```python
from build123d import *

# Parameters (mm, degrees)
EXTRUDE1_DEPTH = 101.6
EXTRUDE2_REACH = 180.036
SKETCH2_R      = 27.805675623


with BuildPart() as part:
    # Sketch1 → Extrude1 (new body)
    with BuildSketch(Plane(origin=(0, 0, 0), x_dir=(1, 0, 0), z_dir=(0, 1, 0))):
        Polygon((0, 36.981224411), (0, 0), (42.615353822, 0), (51.897733448, -10.30089681), (80.325021053, -10.30089681), (89.607400679, 0), (132.222754501, 0), (132.222754501, 36.981224411), align=None)
    extrude(amount=-EXTRUDE1_DEPTH)

    # Sketch2 → Extrude2 (add, up to next)
    with BuildSketch(Plane.XY.offset(25.4), mode=Mode.PRIVATE) as extrude2_sk1:
        with Locations((66.111377251, -50.8)):
            Circle(SKETCH2_R)
    extrude2_tool1 = extrude(extrude2_sk1.sketch, amount=-EXTRUDE2_REACH, mode=Mode.PRIVATE) - part.part
    add(extrude2_tool1.solids().sort_by_distance((66.111377, -50.8, 25.4))[0])


solid = part.part
```
Work out the finished part from the listing and answer in its coordinate system (mm). A direction names the side the tool comes from. Give positions to 0.01 mm unless a question says otherwise; leave off trailing zeros. Loops run counter-clockwise (first coordinate to the right, second up) from the corner with the lowest first, then second, coordinate; pieces in that order, holes last. Notation, with made-up numbers: (55, -9) -> (79, -9) arc R26 cw to (79, 29) -> close; hole circle Ø4 at (-2.5, 50). An arc over 180 degrees is marked (long way). Use CSV: the item, a comma, the result in double quotes.
1. The part is cut by section C-C (x = 117). Write down the section's boundary in (y, z), then the cut area to 3 significant figures.
Found:
outline,"(-101.6, -36.98) -> (0, -36.98) -> (0, 0) -> (-101.6, 0) -> close"
area,"3,760 mm^2"
2. The part is cut by section B-B (z = 15). Write down the section's boundary in (x, y).
Found:
outline,"circle Ø55.61 at (66.11, -50.8)"
3. A tool of negligible diameter and unlimited length cuts with its end or side. For faces 1 (the flat face through (84.901, -87.375, 5.223)), 2 (the flat face through (47.192, -87.375, 5.078)), 3 (the cylindrical face through (38.333, -49.577, 15.7)), from which of +Z, -Z, +X, -X, +Y, -Y can it reach the whole face along a straight path? Write none if from no direction.
Found:
face 1,"+Z, +X, -Y"
face 2,"+Z, -X, -Y"
face 3,"+Z"
4. Flat-ended cylindrical pins translate along their axes: pin 1 Ø13 at (x, y) = (29, -25.5) entering from +Z; pin 2 Ø13.5 at (x, y) = (71.5, -14) entering from +Z. Find the tip coordinate at first contact, or state that the pin passes through.
Found:
pin 1,"z = 0"
pin 2,"z = 10.3"
5. Straight lines are drawn through the part: line 1 (Z direction, x = 54.5, y = -79); line 2 (Z direction, x = 6.5, y = -76); line 3 (X direction, y = -66, z = 19.5). For each, find the intervals that lie inside material, in ascending order.
Found:
line 1,"-36.98 to 10.3"
line 2,"-36.98 to 0"
line 3,"42.83 to 89.39"
6. The part is cut by section D-D (y = -50.8). Write down the section's boundary in (x, z), then the cut area to 3 significant figures.
Found:
outline,"(0, -36.98) -> (132.22, -36.98) -> (132.22, 0) -> (93.92, 0) -> (93.92, 25.4) -> (38.31, 25.4) -> (38.31, 0) -> (0, 0) -> close"
area,"6,300 mm^2"
7. The part is cut by section A-A (y = -94.5). Write down the section's boundary in (x, z).
Found:
outline,"(0, -36.98) -> (132.22, -36.98) -> (132.22, 0) -> (89.61, 0) -> (80.33, 10.3) -> (51.9, 10.3) -> (42.62, 0) -> (0, 0) -> close"
